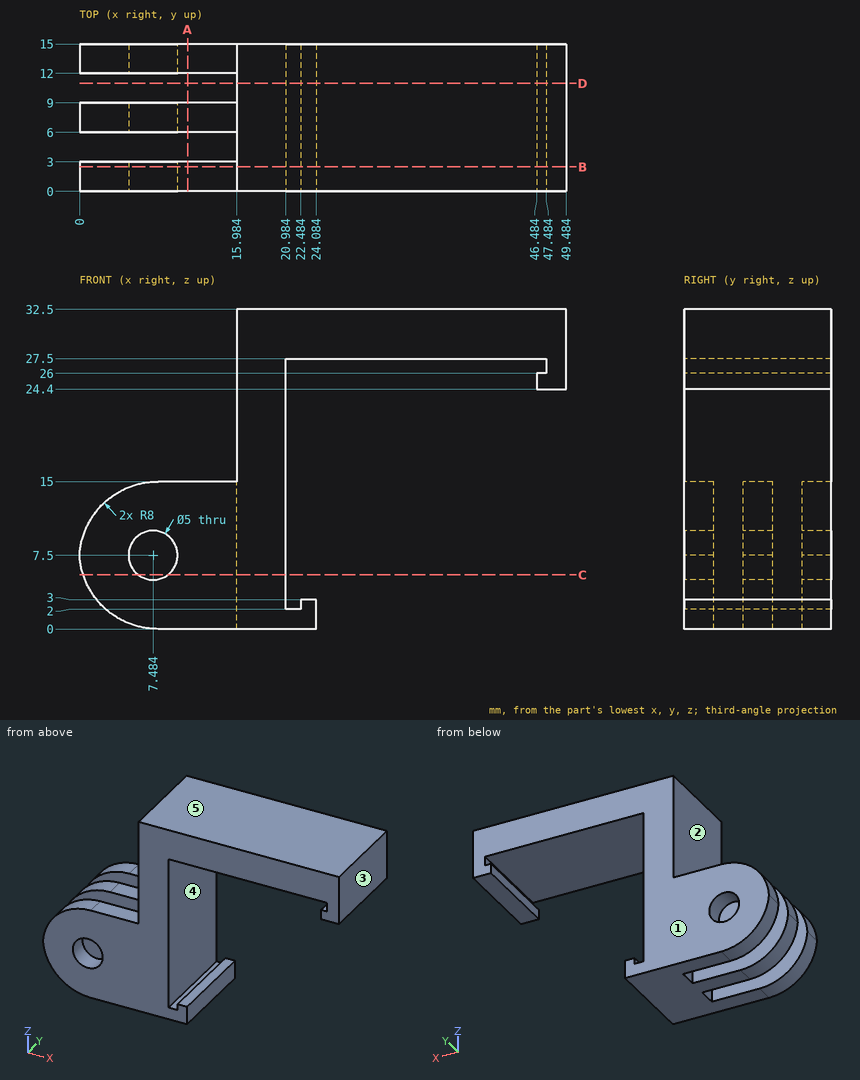
Job drawing, mm, ordinate dimensions from the low corner. One solid piece. A direction names the side the tool comes from. Give positions to 0.01 mm unless a question says otherwise; leave off trailing zeros. Write each loop counter-clockwise with the first axis right and the second up, starting at its lowest first coordinate (ties: lowest second). Pieces come first, ordered by that corner, then holes. Notation, with made-up numbers: M 74,65 L 117,65 A31 cw 117,103 Z; hole C 40.5,29.25 d4. An arc over 180 degrees is marked long. Put each result on its own line as item: value. Start each with the question number.
(1) Flat gauge pins, fed straight in: pin 1 Ø1.5 at (x, y) = (12, 2.5) entering from +Z; pin 2 Ø1.5 at (y, z) = (7.5, 2) entering from +X; pin 3 Ø8 at (y, z) = (11, 10) entering from +X. Where does each tip first touch, or does it go through?
(2) Band-saw the part on B-B, the plane y = 2.5. Write the cut outline in (x, z) (1 decimal).
(3) Band-saw the part on C-C, the plane z = 5.5. Write the cut outline in (x, y) (1 decimal), and give its area (3 significant figures).
(4) Band-saw the part on A-A, the plane x = 11. Write the cut outline in (y, z), and give its area (3 significant figures).
(5) Which spindle directions (+Z, -Z, +X, -X, +Y, -Y) get a long thin tool onto all of the face, cutting with end or side? Do the marked faces 1 and 2. Say none if no direction does.
(6) Probe L1, parallel to Y at x = 9.5, z = 12; L2, parallel to Z at x = 22, y = 6.5; L3, parallel to Z at x = 42, y = 2.75. List the from-to ranges inside material, lowest first.
(7) Mould opens along Z. For the marked faces 3, 4 and 5 say: +Z half, -Z half, draft (parallel to the pull), parting line (faces both ways), or undercut.
(8) Band-saw the part on D-D, the plane y = 11. Write the cut outline in (x, z) (1 decimal).
Response values:
1. pin 1: stops at z = 15
1. pin 2: stops at x = 24.08
1. pin 3: stops at x = 20.98
2. outline: M 0,7.5 A8 ccw 8,0 L 24.1,0 L 24.1,3 L 22.5,3 L 22.5,2 L 21,2 L 21,27.5 L 47.5,27.5 L 47.5,26 L 46.5,26 L 46.5,24.4 L 49.5,24.4 L 49.5,32.5 L 16,32.5 L 16,15 L 8,15 A8 ccw Z; hole C 7.5,7.5 d5
3. outline: M 0.4,0 L 6,0 L 6,3 L 0.4,3 Z; M 0.4,6 L 6,6 L 6,9 L 0.4,9 Z; M 0.4,12 L 6,12 L 6,15 L 0.4,15 Z; M 9,0 L 21,0 L 21,15 L 9,15 L 9,12 L 16,12 L 16,9 L 9,9 L 9,6 L 16,6 L 16,3 L 9,3 Z
3. area: 188 mm2
4. outline: M 0,0 L 3,0 L 3,15 L 0,15 Z; M 6,0 L 9,0 L 9,15 L 6,15 Z; M 12,0 L 15,0 L 15,15 L 12,15 Z
4. area: 135 mm2
5. face 1: +Z, -Z, +X, -X, +Y
5. face 2: +Z, -X
6. L1: y = 0 to 3, 6 to 9, 12 to 15
6. L2: z = 0 to 2, 27.5 to 32.5
6. L3: z = 27.5 to 32.5
7. face 3: draft
7. face 4: undercut
7. face 5: +Z half
8. outline: M 16,0 L 24.1,0 L 24.1,3 L 22.5,3 L 22.5,2 L 21,2 L 21,27.5 L 47.5,27.5 L 47.5,26 L 46.5,26 L 46.5,24.4 L 49.5,24.4 L 49.5,32.5 L 16,32.5 Z
